from build123d import *

# Parameters (mm, degrees)
F0_W          = 80
F0_H          = 50
F0_W_2        = 76
F0_H_2        = 46
F1_DEPTH      = 10
F1_DEPTH_BACK = 10
F2_R          = 2.5
F3_DEPTH      = 40
F3_DEPTH_BACK = 40


with BuildPart() as f1:
    # F0 (on Top) → F1 (new body, two sides)
    with BuildSketch(Plane.XY) as f1_sk:
        Rectangle(F0_W, F0_H)
        Rectangle(F0_W_2, F0_H_2, mode=Mode.SUBTRACT)
    extrude(amount=F1_DEPTH)
    extrude(f1_sk.sketch, amount=-F1_DEPTH_BACK)

    # F2 (on Front) → F3 (cut, two sides)
    with BuildSketch(Plane.XZ) as f3_sk:
        with Locations((-30, 0)):
            Circle(F2_R)
        Circle(F2_R)
        with Locations((30, 0)):
            Circle(F2_R)
    extrude(amount=F3_DEPTH, mode=Mode.SUBTRACT)
    extrude(f3_sk.sketch, amount=-F3_DEPTH_BACK, mode=Mode.SUBTRACT)


solid = f1.part
The model under review builds one solid part; all positions refer to its coordinate system, in mm. A direction names the side the tool comes from. Round coordinates to 2 decimals unless told otherwise and drop trailing zeros. Write each loop counter-clockwise with the first axis right and the second up, starting at its lowest first coordinate (ties: lowest second). Pieces come first, ordered by that corner, then holes. Notation, with made-up numbers: M -0.75,41 L 35.25,41 A12 cw 35.25,48 Z; hole C 45,-12 d7. An arc over 180 degrees is marked long. Use a Markdown table: item, result. Add a question column.
Q1. The part is to be moulded in two halves that separate along Z. For faces 1 (the face through (27.5, 24, 0.1)), 2 (the face through (-1, -23, 5)), 3 (the face through (-3, -24, -10)), say which applies: pulls with the +Z half, pulls with the -Z half, needs draft (parallel to the pull), parting line crosses it, or undercut.
Q2. We need section C-C, the plane y = 1.5. State the section outline as (x, z) points, plus the area to 3 significant figures.
Q3. We need section D-D, the plane z = 0. Count the separate pieces of the cut face and the enclosed holes in it, plus the area to 3 significant figures.
Q4. To check wall thickness, follow line 1 (X direction, y = -24.1, z = 0); line 2 (Y direction, x = 14.5, z = -8); line 3 (X direction, y = -18, z = -6.5). State the ranges of each line that lie inside material, in increasing order.
Q5. Machinability: for faces 4 (the face through (-0.54, 23.99, -2.44)), 5 (the face through (-1, 23, 5)), which of the approach directions +Z, -Z, +X, -X, +Y, -Y give a long, thin tool a straight path to every point of the face, cutting with its end or side? Answer none if there is none.
Q6. We need section B-B, the plane z = 6. State the section outline as (x, y) points.
Q7. We need section A-A, the plane x = 30. State the section outline as (y, z) points.
Findings below:
| question | item | result |
|---|---|---|
| 1 | face 1 | undercut |
| 1 | face 2 | needs draft |
| 1 | face 3 | pulls with the -Z half |
| 2 | outline | M -40,-10 L -38,-10 L -38,10 L -40,10 Z; M 38,-10 L 40,-10 L 40,10 L 38,10 Z |
| 2 | area | 80.0 mm² |
| 3 | separate pieces | 6 |
| 3 | enclosed holes | 0 |
| 3 | area | 444 mm² |
| 4 | line 1 | x = -40 to -32.5, -27.5 to -2.5, 2.5 to 27.5, 32.5 to 40 |
| 4 | line 2 | y = -25 to -23, 23 to 25 |
| 4 | line 3 | x = -40 to -38, 38 to 40 |
| 5 | face 4 | +Y, -Y |
| 5 | face 5 | +Z, -Z |
| 6 | outline | M -40,-25 L 40,-25 L 40,25 L -40,25 Z; hole M -38,-23 L 38,-23 L 38,23 L -38,23 Z |
| 7 | outline | M -25,-10 L -23,-10 L -23,-2.5 L -25,-2.5 Z; M -25,2.5 L -23,2.5 L -23,10 L -25,10 Z; M 23,-10 L 25,-10 L 25,-2.5 L 23,-2.5 Z; M 23,2.5 L 25,2.5 L 25,10 L 23,10 Z |
